Answer from the drawing. Dimensions are ordinates in mm from the lowest x, y and z of the part. Round coordinates to 2 decimals unless told otherwise and drop trailing zeros. Write each loop counter-clockwise with the first axis right and the second up, starting at its lowest first coordinate (ties: lowest second). Pieces come first, ordered by that corner, then holes. Notation, with made-up numbers: (-7, -13.75) - (26, -13.75) arc R22 cw to (26, 15.25) - close; hole circle Ø10 at (69, 32.25). An arc over 180 degrees is marked (long way). Answer as CSV lines item,"result". Start each with the question number.
1) Consider line 1 along Y through (x, z) = (4.25, 6); line 2 along Y through (x, z) = (6.5, 6) (1 decimal); line 3 along X through (y, z) = (15.25, 5.75) (1 decimal). Determine where each line is inside the solid, lowest interval first.
2) Find section B-B on y = 16. Determine the outline of the cut face in (x, z).
3) Each of these flat-tipped pins is pushed along its axis until it touches: pin 1 (1 mm diameter, centred on x = 5.5, z = 2, fed in from +Y); pin 2 (2 mm diameter, centred on y = 14, z = 3, fed in from -X). Where does it stop, or does it pass through?
4) Find section A-A on x = 4.25. Determine the outline of the cut face in (y, z), then the cut area to 3 significant figures.
5) Find section D-D on y = 11. Determine the outline of the cut face in (x, z).
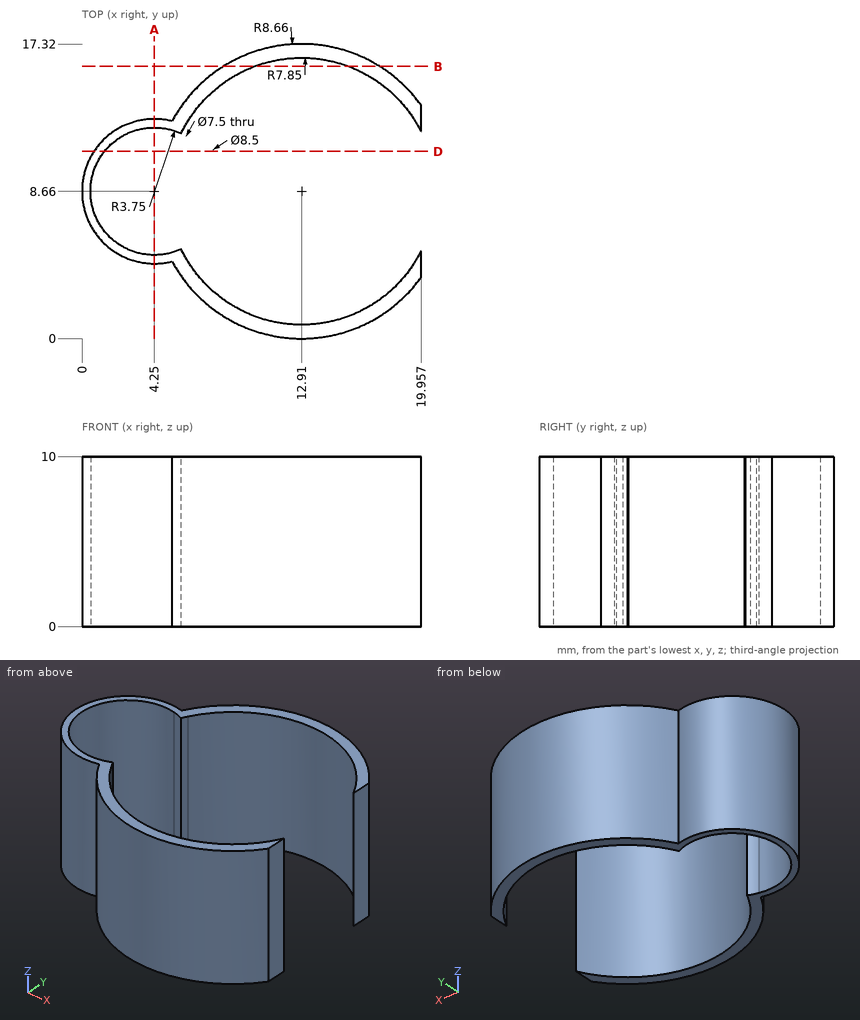
Check values:
1,line 1,"y = 4.41 to 4.91, 12.41 to 12.91"
1,line 2,"y = 2.8 to 4.1, 13.2 to 14.5"
1,line 3,"x = 7.3 to 8.6, 17.2 to 18.5"
2,outline,"(8.31, 0) - (10.13, 0) - (10.13, 10) - (8.31, 10) - close; (15.69, 0) - (17.51, 0) - (17.51, 10) - (15.69, 10) - close"
3,pin 1,"stops at y = 13.88"
3,pin 2,"stops at x = 5.42"
4,outline,"(4.41, 0) - (4.91, 0) - (4.91, 10) - (4.41, 10) - close; (12.41, 0) - (12.91, 0) - (12.91, 10) - (12.41, 10) - close"
4,area,"10.0 mm^2"
5,outline,"(0.7, 0) - (1.32, 0) - (1.32, 10) - (0.7, 10) - close"
